Read the model definition and answer for the solid it produces. Units are mm, in the model's axes. Face numbers are marked on the shaded views. A direction names the side the tool comes from. Round coordinates to 2 decimals unless told otherwise and drop trailing zeros. Loops run counter-clockwise (first coordinate to the right, second up) from the corner with the lowest first, then second, coordinate; pieces in that order, holes last. Notation, with made-up numbers: M 65,80.5 L 76,80.5 A23 cw 76,108.5 Z; hole C 51,-16 d11. An arc over 180 degrees is marked long. Write each question's results on one line, items separated by ' | '.
from build123d import *

# Parameters (mm, degrees)
SKETCH1_W           = 78.03
SKETCH1_H           = 25
BOSS_EXTRUDE1_DEPTH = 21
SKETCH2_R           = 10
BOSS_EXTRUDE2_DEPTH = 40
SKETCH4_R           = 6.25
BOSS_EXTRUDE3_DEPTH = 65.56
CHAMFER1_SIZE       = 5.56


with BuildPart() as part:
    # Sketch1 → Boss-Extrude1 (new body)
    with BuildSketch(Plane.XY):
        Rectangle(SKETCH1_W, SKETCH1_H)
    extrude(amount=-BOSS_EXTRUDE1_DEPTH)

    # Sketch2 → Boss-Extrude2 (add)
    with BuildSketch(Plane(origin=(39.015, 0, 0), x_dir=(0, 0, -1), z_dir=(1, 0, 0))):
        with Locations((10.5, 0)):
            Circle(SKETCH2_R)
    extrude(amount=BOSS_EXTRUDE2_DEPTH)

    # Sketch4 → Boss-Extrude3 (add)
    with BuildSketch(Plane(origin=(0, 0, -21), x_dir=(-1, 0, 0), z_dir=(0, 0, -1))):
        with Locations((-6.565, 0)):
            Circle(SKETCH4_R)
    extrude(amount=BOSS_EXTRUDE3_DEPTH)

    # Chamfer1
    chamfer1_edges = [part.edges().sort_by_distance(p)[0] for p in [
        (12.815, 0, -86.56),
    ]]
    chamfer(chamfer1_edges, length=CHAMFER1_SIZE)


solid = part.part
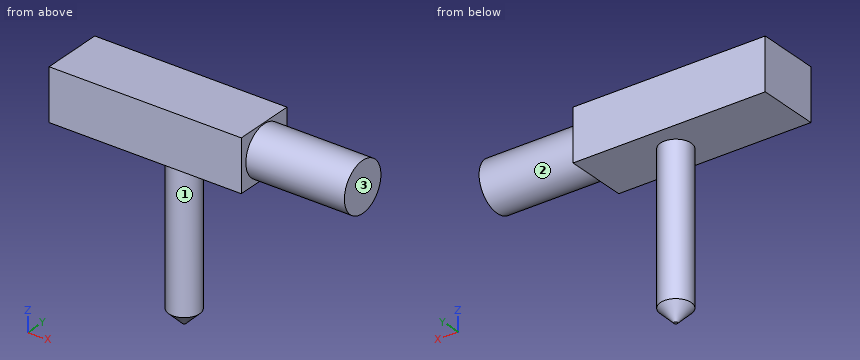
Item 1: The part is cut by section B-B (y = -8.5). Determine the outline of the cut face in (x, z) (3 decimals), plus the area to 3 significant figures.
Outcome:
outline: M -39.015,-21 L 39.015,-21 L 39.015,-15.768 L 79.015,-15.768 L 79.015,-5.232 L 39.015,-5.232 L 39.015,0 L -39.015,0 Z | area: 2,060 mm2
Item 2: Flat-ended cylindrical pins translate along their axes: pin 1 (8 mm diameter, centred on y = 4, z = -43, fed in from +X) (3 decimals); pin 2 (5 mm diameter, centred on x = 30, y = 8, fed in from -Z); pin 3 (3 mm diameter, centred on x = -3, z = -36, fed in from -Y); pin 4 (1 mm diameter, centred on y = 0, z = -37, fed in from -X) (3 decimals). Find the tip coordinate at first contact, or state that the pin passes through.
Outcome:
pin 1: stops at x = 12.815 | pin 2: stops at z = -21 | pin 3: passes through | pin 4: stops at x = 0.315
Item 3: The part is cut by section C-C (x = 41). Determine the outline of the cut face in (y, z).
Outcome:
outline: C 0,-10.5 d20
Item 4: The part is cut by section A-A (z = -10.5). Determine the outline of the cut face in (x, y) (3 decimals).
Outcome:
outline: M -39.015,-12.5 L 39.015,-12.5 L 39.015,-10 L 79.015,-10 L 79.015,10 L 39.015,10 L 39.015,12.5 L -39.015,12.5 Z
Item 5: For the marked faces 1, 2 and 3, determine the directions among +Z, -Z, +X, -X, +Y, -Y from which every point of the face is accessible in a straight line to the end or side of a thin tool.
Outcome:
face 1: -Z | face 2: +X | face 3: +Z, -Z, +X, +Y, -Y
Item 6: The part is cut by section D-D (z = -23.5). Determine the outline of the cut face in (x, y) (3 decimals).
Outcome:
outline: C 6.565,0 d12.5
Item 7: Straight lines are drawn through the part: line 1 (Z direction, x = -30, y = 8); line 2 (Y direction, x = 7, z = -32); line 3 (X direction, y = 8.75, z = -20) (3 decimals). For each, find the intervals that lie inside material, in ascending order.
Outcome:
line 1: z = -21 to 0 | line 2: y = -6.23 to 6.23 | line 3: x = -39.015 to 39.015
